Read the model definition and answer for the solid it produces. Units are mm, in the model's axes. A direction names the side the tool comes from. Coordinates: 2 decimals unless noted, no trailing zeros. Write each loop counter-clockwise with the first axis right and the second up, starting at its lowest first coordinate (ties: lowest second). Pieces come first, ordered by that corner, then holes.
1) The part is cut by section C-C (z = 1.75). Determine the outline of the cut face in (x, y), then the cut area to 3 significant figures.
2) The part is cut by section D-D (z = 0). Determine the outline of the cut face in (x, y), then the cut area to 3 significant figures.
3) The part is cut by section A-A (x = 0). Determine the outline of the cut face in (y, z), then the cut area to 3 significant figures.
4) Determine the mould class of faces 1 (the face through (-13.735, 4.325, -2.268)), 2 (the face through (3.47, -15.62, -0.04)), 3 (the face through (-7.8, 12.3, 3.5)) for opening direction X: +X half, -X half, draft (parallel to the pull), parting line (faces both ways), or undercut.
5) Each of these flat-tipped pins is pushed along its axis until it touches: pin 1 Ø8.5 at (x, y) = (5.5, 0) entering from -Z; pin 2 Ø1 at (y, z) = (-1, -2.5) entering from -X; pin 3 Ø5 at (x, y) = (-9, 7.5) entering from +Z. Where does it stop, or does it pass through?
6) Find the intervals of material crossed by line 1 (Y direction, x = 0, z = -1.6); line 2 (Z direction, x = -3, y = 4); line 3 (Y direction, x = 10, z = 2.75), in increasing order.
7) Which of the six approach directions +Z, -Z, +X, -X, +Y, -Y give full straight-line access (tool end or side, diameter ignored) to faces 4 (the face through (-13.735, 4.325, 2.268)), 5 (the face through (-7.8, 12.3, -3.5)), 6 (the face through (0, 0, -1))?
from build123d import *

# Parameters (mm, degrees)
F3_R = 1
F4_R = 1


with BuildPart() as f1:
    # F0 (on Front) → F1 (revolve)
    with BuildSketch(Plane.XZ):
        Polygon((-16, 0), (0, 0), (0, 1), (-14.4, 1), (-14.4, 3.5), (-16, 3.5), align=None)
    revolve(axis=Axis((0, 0, -1.1237002909), (0, 0, -1)))

    # F2: F1 across plane


with BuildPart() as f1_1:
    add(f1.part)
    add(f1.part.mirror(Plane.XY))

    # F3
    f3_edges = [f1_1.edges().sort_by_distance(p)[0] for p in [
        (16, 0, 3.5),
    ]]
    fillet(f3_edges, radius=F3_R)

    # F4
    f4_edges = [f1_1.edges().sort_by_distance(p)[0] for p in [
        (16, 0, -3.5),
    ]]
    fillet(f4_edges, radius=F4_R)


solid = f1_1.part
Reported:
1. outline: circle Ø32 at (0, 0); hole circle Ø28.8 at (0, 0)
1. area: 153 mm2
2. outline: circle Ø32 at (0, 0)
2. area: 804 mm2
3. outline: (-16, -2.5) arc R1 ccw to (-15, -3.5) - (-14.4, -3.5) - (-14.4, -1) - (14.4, -1) - (14.4, -3.5) - (15, -3.5) arc R1 ccw to (16, -2.5) - (16, 2.5) arc R1 ccw to (15, 3.5) - (14.4, 3.5) - (14.4, 1) - (-14.4, 1) - (-14.4, 3.5) - (-15, 3.5) arc R1 ccw to (-16, 2.5) - close
3. area: 79.1 mm2
4. face 1: undercut
4. face 2: parting line
4. face 3: draft
5. pin 1: stops at z = -1
5. pin 2: stops at x = -15.99
5. pin 3: stops at z = 1
6. line 1: y = -16 to -14.4, 14.4 to 16
6. line 2: z = -1 to 1
6. line 3: y = -12.45 to -10.36, 10.36 to 12.45
7. face 4: +Z
7. face 5: -Z, +X, -X, +Y, -Y
7. face 6: -Z
